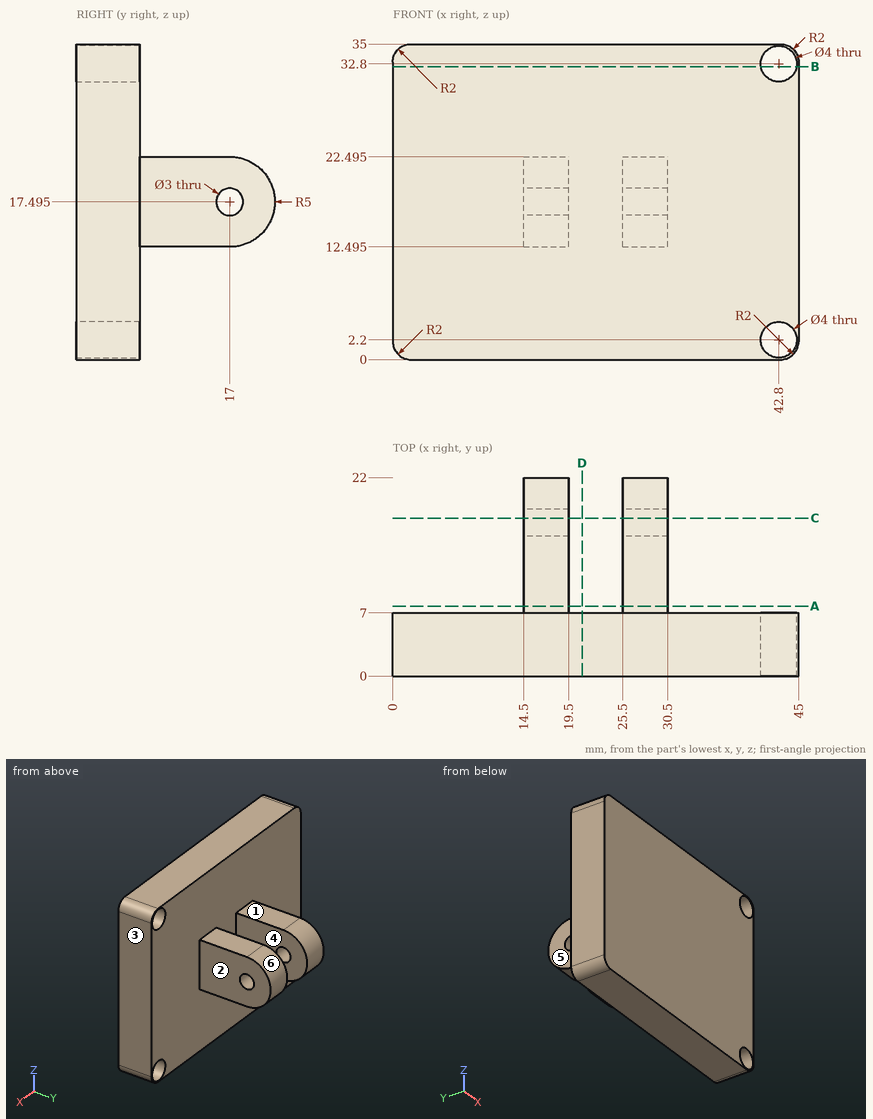
The figure shows three views and two pictorial views of one solid part (mm, origin at its lowest corner). Answer the questions. A direction names the side the tool comes from. Coordinates: 2 decimals unless noted, no trailing zeros. Loops run counter-clockwise (first coordinate to the right, second up) from the corner with the lowest first, then second, coordinate; pieces in that order, holes last.
(1) A tool of negligible diameter and unlimited length cuts with its end or side. For the marked faces 1, 2 and 3, from which of +Z, -Z, +X, -X, +Y, -Y can it reach the whole face along a straight path? Write none if from no direction.
Solution:
face 1: +Z, +X, -X, +Y
face 2: +Z, -Z, +X, +Y
face 3: +Z, -Z, +X, +Y, -Y
(2) The part is cut by section A-A (y = 7.75). Determine the outline of the cut face in (x, z) (3 decimals), and give its area (3 significant figures).
Solution:
outline: (14.5, 12.495) - (19.5, 12.495) - (19.5, 22.495) - (14.5, 22.495) - close; (25.5, 12.495) - (30.5, 12.495) - (30.5, 22.495) - (25.5, 22.495) - close
area: 100 mm2
(3) Flat-ended cylindrical pins translate along their axes: pin 1 Ø5 at (y, z) = (18, 18.5) entering from -X; pin 2 Ø5 at (x, z) = (42.8, 2.2) entering from +Y; pin 3 Ø1.5 at (x, y) = (18, 10.5) entering from +Z (3 decimals). Find the tip coordinate at first contact, or state that the pin passes through.
Solution:
pin 1: stops at x = 14.5
pin 2: stops at y = 7
pin 3: stops at z = 22.495
(4) The part is cut by section C-C (y = 17.5). Determine the outline of the cut face in (x, z).
Solution:
outline: (14.5, 12.52) - (19.5, 12.52) - (19.5, 16.08) - (14.5, 16.08) - close; (14.5, 18.91) - (19.5, 18.91) - (19.5, 22.47) - (14.5, 22.47) - close; (25.5, 12.52) - (30.5, 12.52) - (30.5, 16.08) - (25.5, 16.08) - close; (25.5, 18.91) - (30.5, 18.91) - (30.5, 22.47) - (25.5, 22.47) - close
(5) The mould has two halves that part along X. Classify the marked faces 4, 5 and 6: released by +X, released by -X, zero draft, split by the parting line, or undercut.
Solution:
face 4: undercut
face 5: released by -X
face 6: zero draft
(6) The part is cut by section B-B (z = 32.5). Determine the outline of the cut face in (x, y), and give its area (3 significant figures).
Solution:
outline: (0, 0) - (40.82, 0) - (40.82, 7) - (0, 7) - close; (44.78, 0) - (45, 0) - (45, 7) - (44.78, 7) - close
area: 287 mm2
(7) The part is cut by section D-D (x = 21). Determine the outline of the cut face in (y, z).
Solution:
outline: (0, 0) - (7, 0) - (7, 35) - (0, 35) - close
(8) Consider line 1 along X through (y, z) = (15, 13.5); line 2 along Y through (x, z) = (15, 17.5); line 3 along X through (y, z) = (5.5, 32.8). Determine where each line is inside the solid, lowest interval first.
Solution:
line 1: x = 14.5 to 19.5, 25.5 to 30.5
line 2: y = 0 to 15.5, 18.5 to 22
line 3: x = 0 to 40.8, 44.8 to 45
